The model under review builds one solid part; all positions refer to its coordinate system, in mm. Face numbers are marked on the shaded views. A direction names the side the tool comes from. Coordinates: 2 decimals unless noted, no trailing zeros. Loops run counter-clockwise (first coordinate to the right, second up) from the corner with the lowest first, then second, coordinate; pieces in that order, holes last. Notation, with made-up numbers: M -34.5,58.5 L -9.5,58.5 A14 ccw -9.5,69.5 Z; hole C 88,66.25 d11. An arc over 180 degrees is marked long. Use one line per item in the form item = value.
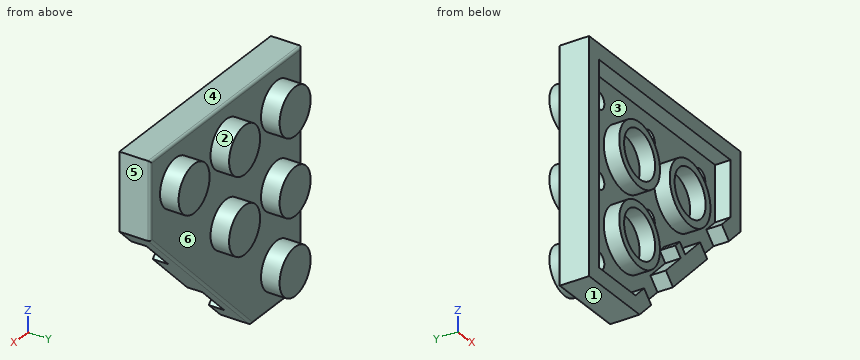
```python
from build123d import *

# Parameters (mm, degrees)
SKETCH1_W                = 23.8125
SKETCH1_H                = 23.8125
BASE_EXTRUDE_DEPTH       = 3.175
SKETCH2_R                = 2.4384
BOSS_EXTRUDE1_DEPTH      = 1.905
LPATTERN4_COUNT          = 3
LPATTERN4_PITCH          = 7.9375
LPATTERN4_COUNT_DIR2     = 3
LPATTERN4_PITCH_DIR2     = 7.9375
CUT_EXTRUDE1_DEPTH       = 18.134707559
SHELL1_T                 = -1.5875
SKETCH3_R                = 3.2004
SKETCH3_R_2              = 2.4384
INSDOT_DEPTH             = 1.5875
SKETCH5_R                = 3.2004
SKETCH5_R_2              = 2.4384
BOSS_EXTRUDE_THIN1_DEPTH = 1.5875
SKETCH6_R                = 3.2004
SKETCH6_R_2              = 2.4384
BOSS_EXTRUDE_THIN2_DEPTH = 1.5875
CUT_EXTRUDE2_START       = -1.5875
CUT_EXTRUDE2_DEPTH       = 1.5875
BOSS_EXTRUDE_THIN3_REACH = 19.588
FILLET1_R                = 0.254


with BuildPart() as part:
    # Sketch1 → Base-Extrude (new body)
    with BuildSketch(Plane(origin=(0, 0, 0), x_dir=(1, 0, 0), z_dir=(0, 1, 0))):
        Rectangle(SKETCH1_W, SKETCH1_H)
    extrude(amount=BASE_EXTRUDE_DEPTH)

    # Sketch2 → Boss-Extrude1 (add)
    with BuildSketch(Plane(origin=(0, 3.175, 0), x_dir=(-1, 0, 0), z_dir=(0, 1, 0))):
        with Locations(Location((7.9375, 7.9375, 0), (0, 0, 270))):
            Circle(SKETCH2_R)
    boss_extrude1 = extrude(amount=BOSS_EXTRUDE1_DEPTH)

    # LPattern4: Boss-Extrude1 3 × 3, 3 skipped
    with Locations(*[(i * LPATTERN4_PITCH, 0, -j * LPATTERN4_PITCH_DIR2) for i in range(LPATTERN4_COUNT) for j in range(LPATTERN4_COUNT_DIR2) if (i, j) not in ((0, 0), (1, 2), (2, 1), (2, 2))]):
        add(boss_extrude1)

    # Sketch4 → Cut-Extrude1 (cut, through all)
    with BuildSketch(Plane(origin=(0, 3.175, 0), x_dir=(-1, 0, 0), z_dir=(0, 1, 0))):
        Polygon((-11.90625, 3.96875), (3.96875, -11.90625), (-11.90625, -11.90625), align=None)
    extrude(amount=-CUT_EXTRUDE1_DEPTH, mode=Mode.SUBTRACT)

    # Shell1
    shell1_openings = [part.faces().sort_by_distance(p)[0] for p in [
        (-1.889880952, 0, 1.889880952),
    ]]
    offset(amount=SHELL1_T, openings=shell1_openings, kind=Kind.INTERSECTION)

    # Sketch3 → InsDot (add)
    with BuildSketch(Plane.XZ.offset(-1.5875)):
        with Locations((-3.96875, -3.96875)):
            Circle(SKETCH3_R)
        with Locations((-3.96875, -3.96875)):
            Circle(SKETCH3_R_2, mode=Mode.SUBTRACT)
    extrude(amount=INSDOT_DEPTH)

    # Sketch5 → Boss-Extrude-Thin1 (add)
    with BuildSketch(Plane(origin=(-0.918447423, 1.5875, 6.872038401), x_dir=(1, 0, 0), z_dir=(0, -1, 0))):
        with Locations((-3.050302577, -2.903288401)):
            Circle(SKETCH5_R)
        with Locations((-3.050302577, -2.903288401)):
            Circle(SKETCH5_R_2, mode=Mode.SUBTRACT)
    extrude(amount=BOSS_EXTRUDE_THIN1_DEPTH)

    # Sketch6 → Boss-Extrude-Thin2 (add)
    with BuildSketch(Plane(origin=(7.701488358, 1.5875, 8.898864744), x_dir=(1, 0, 0), z_dir=(0, -1, 0))):
        with Locations((-3.732738358, -4.930114744)):
            Circle(SKETCH6_R)
        with Locations((-3.732738358, -4.930114744)):
            Circle(SKETCH6_R_2, mode=Mode.SUBTRACT)
    extrude(amount=BOSS_EXTRUDE_THIN2_DEPTH)

    # Sketch7 → Cut-Extrude2 (cut)
    with BuildSketch(Plane.XZ.offset(CUT_EXTRUDE2_START)):
        Polygon((5.540294821, -0.152141149), (6.662826836, -1.274673164), (10.075324162, 2.137824162), (8.952792147, 3.260356177), align=None)
        Polygon((-3.260356177, -8.952792147), (0.152141149, -5.540294821), (1.274673164, -6.662826836), (-2.137824162, -10.075324162), align=None)
    extrude(amount=CUT_EXTRUDE2_DEPTH, mode=Mode.SUBTRACT)

    # Sketch8 → Boss-Extrude-Thin3 (add, up to next)
    with BuildSketch(Plane.XZ, mode=Mode.PRIVATE) as boss_extrude_thin3_sk1:
        Polygon((3.241680915, -2.534574133), (2.343655303, -1.636548521), (1.636548521, -2.343655303), (2.534574133, -3.241680915), align=None)
    boss_extrude_thin3_tool1 = extrude(boss_extrude_thin3_sk1.sketch, amount=-BOSS_EXTRUDE_THIN3_REACH, mode=Mode.PRIVATE) - part.part
    add(boss_extrude_thin3_tool1.solids().sort_by_distance((2.439115, 0, -2.439115))[0])

    # Fillet1
    fillet1_edges = [part.edges().sort_by_distance(p)[0] for p in [
        (11.90625, 3.175, 7.9375),
        (-7.9375, 3.175, -11.90625),
        (3.96875, 3.175, -3.96875),
        (-11.90625, 3.175, 0),
        (0, 3.175, 11.90625),
    ]]
    fillet(fillet1_edges, radius=FILLET1_R)


solid = part.part
```
1. Add section B-B (y = 4.3). State the section outline as (x, z) points, then the cut area to 3 significant figures.
Response values:
outline = C -7.94,-7.94 d4.88; C -7.94,0 d4.88; C -7.94,7.94 d4.88; C 0,0 d4.88; C 0,7.94 d4.88; C 7.94,7.94 d4.88
area = 112 mm^2
2. Add section A-A (y = 1.3). State the section outline as (x, z) points.
Response values:
outline = M -11.91,-11.91 L -3.97,-11.91 L -2.14,-10.08 L -3.26,-8.95 L -4.63,-10.32 L -10.32,-10.32 L -10.32,10.32 L 10.32,10.32 L 10.32,4.63 L 8.95,3.26 L 10.08,2.14 L 11.91,3.97 L 11.91,11.91 L -11.91,11.91 Z; C -3.97,-3.97 d6.4; C -3.97,3.97 d6.4; M 0.15,-5.54 L 1.27,-6.66 L 6.66,-1.27 L 5.54,-0.15 L 3.2,-2.49 L 2.34,-1.64 L 1.64,-2.34 L 2.49,-3.2 Z; C 3.97,3.97 d6.4; hole C -3.97,-3.97 d4.88; hole C -3.97,3.97 d4.88; hole C 3.97,3.97 d4.88
3. Wall thickness on line 1 along X through (y, z) = (3.65, 8); line 2 along X through (y, z) = (3, 0); line 3 along Z through (x, y) = (4, 0.8): over which ranges is each line inside the solid? List them lowest first. Write a range as from..to.
Response values:
line_1 = -10.38..-5.5, -2.44..2.44, 5.5..10.38
line_2 = -11.89..-8.79, -7.09..-0.85, 0.85..7.92
line_3 = -3.94..-1.69, 0.77..1.53, 6.41..7.17, 10.32..11.91
4. Machinability: for the marked faces 1, 2 and 3, which of the approach directions +Z, -Z, +X, -X, +Y, -Y give a long, thin tool a straight path to every point of the face, cutting with its end or side? Answer none if there is none.
Response values:
face_1 = -Z, +X, -X, +Y, -Y
face_2 = +Y
face_3 = -Y
5. Insertion check: P1, Ø2.5, axis at x = 0, z = 7.94, coming from the -Y side; P2, Ø1.4, axis at x = 0, z = 0, coming from the -Y side; P3, Ø3, axis at y = 1.5, z = 1, coming from the +X side. Each pin has a flat end and moves straight along its axis. Give the tip position at first contact, or say it passes through.
Response values:
P1 = 1.59
P2 = 3.49
P3 = 10.44
6. The part is to be moulded in two halves that separate along X. For the marked faces 4, 5 and 6, say which applies: pulls with the +X half, pulls with the -X half, needs draft (parallel to the pull), parting line crosses it, or undercut.
Response values:
face_4 = needs draft
face_5 = pulls with the +X half
face_6 = undercut
